from build123d import *

# Parameters (mm, degrees)
SKETCH1_W           = 15.3
SKETCH1_H           = 30
BOSS_EXTRUDE1_DEPTH = 13.1
SKETCH2_R           = 6
BOSS_EXTRUDE2_DEPTH = 10.5
SKETCH4_R           = 5
CUT_EXTRUDE1_DEPTH  = 4
SKETCH5_R           = 3
BOSS_EXTRUDE3_DEPTH = 21.5
REVOLVE2_ANGLE      = 180
FILLET1_R           = 2
SKETCH6_W           = 15.3
SKETCH6_H           = 27
BOSS_EXTRUDE4_DEPTH = 5.2


with BuildPart() as part:
    # Sketch1 → Boss-Extrude1 (new body)
    with BuildSketch(Plane(origin=(0, 0, 0), x_dir=(1, 0, 0), z_dir=(0, 1, 0))):
        Rectangle(SKETCH1_W, SKETCH1_H)
    extrude(amount=BOSS_EXTRUDE1_DEPTH)

    # Sketch2 → Boss-Extrude2 (add)
    with BuildSketch(Plane(origin=(0, 13.1, 0), x_dir=(1, 0, 0), z_dir=(0, 1, 0))):
        Circle(SKETCH2_R)
    extrude(amount=BOSS_EXTRUDE2_DEPTH)

    # Sketch4 → Cut-Extrude1 (cut)
    with BuildSketch(Plane(origin=(0, 23.6, 0), x_dir=(1, 0, 0), z_dir=(0, 1, 0))):
        Circle(SKETCH4_R)
    extrude(amount=-CUT_EXTRUDE1_DEPTH, mode=Mode.SUBTRACT)

    # Sketch5 → Boss-Extrude3 (add)
    with BuildSketch(Plane(origin=(0, 19.6, 0), x_dir=(1, 0, 0), z_dir=(0, 1, 0))):
        Circle(SKETCH5_R)
    extrude(amount=BOSS_EXTRUDE3_DEPTH)

    # Sketch3 → Revolve2 (revolve)
    with BuildSketch(Plane(origin=(0, 19.6, 0), x_dir=(1, 0, 0), z_dir=(0, 1, 0))):
        with BuildLine():
            Line((0, -5), (0, 5))
            ThreePointArc((0, 5), (-5, 0), (0, -5))
        make_face()
    revolve(axis=Axis((0, 19.6, 6), (0, 0, -1)), revolution_arc=REVOLVE2_ANGLE)

    # Fillet1
    fillet1_edges = [part.edges().sort_by_distance(p)[0] for p in [
        (-3, 41.1, 0),
    ]]
    fillet(fillet1_edges, radius=FILLET1_R)

    # Sketch6 → Boss-Extrude4 (add)
    with BuildSketch(Plane.XZ):
        Rectangle(SKETCH6_W, SKETCH6_H)
    extrude(amount=BOSS_EXTRUDE4_DEPTH)


solid = part.part
Could you check a few things on this model? Use its own coordinates, in mm. A direction names the side the tool comes from. Coordinates: 2 decimals unless noted, no trailing zeros. Loops run counter-clockwise (first coordinate to the right, second up) from the corner with the lowest first, then second, coordinate; pieces in that order, holes last.
1. Imagine slicing it at B-B (z = -3.5). Please give me the cut outline in (x, y).
2. For P1, Ø5, axis at x = 0.5, y = 20.5, coming from the +Z side; P2, Ø2, axis at y = 22.5, z = -1.5, coming from the -X side; P3, Ø4, axis at x = 1, y = 33.5, coming from the -Z side, each with a flat end and sliding along its axis, tell me the tip position at first contact or that it passes through.
3. Imagine slicing it at A-A (y = 20.5). Please give me the cut outline in (x, z), and give its area (3 significant figures).
4. I need wall thicknesses on L1, parallel to X at y = 22.2, z = 0; L2, parallel to Z at x = 0, y = 20.85; L3, parallel to X at y = 21, z = 0.75. Which ranges of each line are inside material? Lowest first, please.
5. Imagine slicing it at D-D (z = -8.75). Please give me the cut outline in (x, y), and give its area (3 significant figures).
6. Imagine slicing it at C-C (x = -5.5). Please give me the cut outline in (y, z).
7. For faces 5 (the face through (0, -3, -13.5)), 6 (the face through (-6, 18, 0)), 7 (the face through (0, 6, 15)), 8 (the face through (0, 0, 14)), 9 (the face through (0, -5.2, 0)), which set-ups out of +Z, -Z, +X, -X, +Y, -Y let a thin tool reach every point of the face, with its end or its side?
8. We'd pull the mould along Z, two halves only. Please class faces 1 (the face through (0, 6, -15)), 2 (the face through (0, -3, 13.5)), 3 (the face through (0, 0, -14)), 4 (the face through (-1.08, 21.63, 4.88)): released by +Z, released by -Z, zero draft, split by the parting line, or undercut.
Computed values:
1. outline: (-7.65, -5.2) - (7.65, -5.2) - (7.65, 13.1) - (4.87, 13.1) - (4.87, 23.6) - (3.57, 23.6) - (3.57, 19.6) arc R3.57 ccw to (-3.57, 19.6) - (-3.57, 23.6) - (-4.87, 23.6) - (-4.87, 13.1) - (-7.65, 13.1) - close
2. P1: stops at z = 6
2. P2: stops at x = -5.98
2. P3: stops at z = -3
3. outline: circle Ø12 at (0, 0); circle Ø9.84 at (0, 0); hole circle Ø10 at (0, 0)
3. area: 111 mm2
4. L1: x = -6 to -5, -4.27 to 4.27, 5 to 6
4. L2: z = -6 to -5, -4.84 to 4.84, 5 to 6
4. L3: x = -5.95 to -4.94, -4.74 to 4.74, 4.94 to 5.95
5. outline: (-7.65, -5.2) - (7.65, -5.2) - (7.65, 13.1) - (-7.65, 13.1) - close
5. area: 280 mm2
6. outline: (-5.2, -13.5) - (0, -13.5) - (0, -15) - (13.1, -15) - (13.1, -2.4) - (23.6, -2.4) - (23.6, 2.4) - (13.1, 2.4) - (13.1, 15) - (0, 15) - (0, 13.5) - (-5.2, 13.5) - close
7. face 5: -Z, +X, -X, -Y
7. face 6: +Y
7. face 7: +Z, +X, -X, +Y, -Y
7. face 8: +Z, +X, -X, -Y
7. face 9: +Z, -Z, +X, -X, -Y
8. face 1: released by -Z
8. face 2: released by +Z
8. face 3: zero draft
8. face 4: undercut
